For this review, take the finished solid that the model builds, in its own axes (mm). Round coordinates to 2 decimals unless told otherwise and drop trailing zeros. Write each loop counter-clockwise with the first axis right and the second up, starting at its lowest first coordinate (ties: lowest second). Pieces come first, ordered by that corner, then holes.
from build123d import *

# Parameters (mm, degrees)
SKETCH_1_R          = 50
SKETCH_1_R_2        = 32.5
EXTRUDE_1_DEPTH     = 20
SKETCH_2_R          = 3.2
CUT_EXTRUDE_1_DEPTH = 20


with BuildPart() as part:
    # 草图1 → 凸台-拉伸1 (new body)
    with BuildSketch(Plane(origin=(0, 0, 0), x_dir=(1, 0, 0), z_dir=(0, 1, 0))):
        with Locations(Location((0, 0, 0), (0, 0, 270))):
            Circle(SKETCH_1_R)
        with Locations(Location((0, 0, 0), (0, 0, 270))):
            Circle(SKETCH_1_R_2, mode=Mode.SUBTRACT)
    extrude(amount=EXTRUDE_1_DEPTH)

    # 草图2 → 切除-拉伸1 (cut)
    with BuildSketch(Plane(origin=(0, 20, 0), x_dir=(1, 0, 0), z_dir=(0, 1, 0))):
        with Locations(Location((0, 40, 0), (0, 0, 270))):
            Circle(SKETCH_2_R)
        with Locations(Location((28.284271247, 28.284271247, 0), (0, 0, 270))):
            Circle(SKETCH_2_R)
        with Locations(Location((40, 0, 0), (0, 0, 270))):
            Circle(SKETCH_2_R)
        with Locations(Location((28.284271247, -28.284271247, 0), (0, 0, 270))):
            Circle(SKETCH_2_R)
        with Locations(Location((0, -40, 0), (0, 0, 270))):
            Circle(SKETCH_2_R)
        with Locations(Location((-28.284271247, -28.284271247, 0), (0, 0, 270))):
            Circle(SKETCH_2_R)
        with Locations(Location((-40, 0, 0), (0, 0, 270))):
            Circle(SKETCH_2_R)
        with Locations(Location((-28.284271247, 28.284271247, 0), (0, 0, 270))):
            Circle(SKETCH_2_R)
    extrude(amount=-CUT_EXTRUDE_1_DEPTH, mode=Mode.SUBTRACT)


solid = part.part
(1) We need section B-B, the plane z = 0. Give the boundary of the cut face in (x, y).
Geometry check:
outline: (-50, 0) - (-43.2, 0) - (-43.2, 20) - (-50, 20) - close; (-36.8, 0) - (-32.5, 0) - (-32.5, 20) - (-36.8, 20) - close; (32.5, 0) - (36.8, 0) - (36.8, 20) - (32.5, 20) - close; (43.2, 0) - (50, 0) - (50, 20) - (43.2, 20) - close
(2) We need section A-A, the plane x = -40. Give the boundary of the cut face in (y, z).
Geometry check:
outline: (0, -30) - (20, -30) - (20, -3.2) - (0, -3.2) - close; (0, 3.2) - (20, 3.2) - (20, 30) - (0, 30) - close
(3) For pin 1 Ø5 at (x, y) = (-13, 8) entering from -Z; pin 2 Ø5 at (x, z) = (0, -40) entering from +Y; pin 3 Ø12 at (x, y) = (19, 13) entering from -Z; pin 4 Ø2 at (x, y) = (-25.5, 15) entering from -Z, all flat-tipped, find the tip position at first contact; note any pin that passes through.
Geometry check:
pin 1: stops at z = -48.89
pin 2: passes through
pin 3: stops at z = -48.28
pin 4: stops at z = -43.59
(4) Mouldability with a two-part tool opening along Z and no side actions: class faces 1 (the face through (2.16, 10.14, 37.64)), 2 (the face through (1, 20, 33)), 3 (the face through (15.02, 9.86, 47.69)), 4 (the face through (25.16, 10.14, 27.59)) as pulls with the +Z half, pulls with the -Z half, needs draft (parallel to the pull), parting line crosses it, or undercut.
Geometry check:
face 1: undercut
face 2: needs draft
face 3: parting line crosses it
face 4: undercut
(5) We need section C-C, the plane x = 0. Give the boundary of the cut face in (y, z), and give its area (3 significant figures).
Geometry check:
outline: (0, -50) - (20, -50) - (20, -43.2) - (0, -43.2) - close; (0, -36.8) - (20, -36.8) - (20, -32.5) - (0, -32.5) - close; (0, 32.5) - (20, 32.5) - (20, 36.8) - (0, 36.8) - close; (0, 43.2) - (20, 43.2) - (20, 50) - (0, 50) - close
area: 444 mm2
(6) For line 1 along X through (y, z) = (7.5, 0); line 2 along Z through (x, y) = (30, 15); line 3 along Z through (x, y) = (29, 8.75), list the stretches that pass through material, from the lowest coordinate up.
Geometry check:
line 1: x = -50 to -43.2, -36.8 to -32.5, 32.5 to 36.8, 43.2 to 50
line 2: z = -40 to -30.99, -25.58 to -12.5, 12.5 to 25.58, 30.99 to 40
line 3: z = -40.73 to -31.4, -25.17 to -14.67, 14.67 to 25.17, 31.4 to 40.73
(7) We need section D-D, the plane z = 40. Give the boundary of the cut face in (x, y).
Geometry check:
outline: (-30, 0) - (-3.2, 0) - (-3.2, 20) - (-30, 20) - close; (3.2, 0) - (30, 0) - (30, 20) - (3.2, 20) - close
